from build123d import *

# Parameters (mm, degrees)
F0_R     = 1.1684
F1_DEPTH = 1.1811
F3_DEPTH = 4.7244
F5_DEPTH = 3.4798
F7_DEPTH = 4.4069


with BuildPart() as f1:
    # F0 (on Top) → F1 (new body, symmetric)
    with BuildSketch(Plane.XY):
        with BuildLine():
            Line((16.6497, 4.4577), (-16.6497, 4.4577))
            ThreePointArc((-16.6497, 4.4577), (-17.763252, 3.996452), (-18.2245, 2.8829))
            Line((-18.2245, 2.8829), (-18.2245, -2.8829))
            ThreePointArc((-18.2245, -2.8829), (-17.763252, -3.996452), (-16.6497, -4.4577))
            Line((-16.6497, -4.4577), (16.6497, -4.4577))
            ThreePointArc((16.6497, -4.4577), (17.763252, -3.996452), (18.2245, -2.8829))
            Line((18.2245, -2.8829), (18.2245, 2.8829))
            ThreePointArc((18.2245, 2.8829), (17.763252, 3.996452), (16.6497, 4.4577))
        make_face()
        with Locations((-15.4305, 0)):
            Circle(F0_R, mode=Mode.SUBTRACT)
        with Locations((15.4305, 0)):
            Circle(F0_R, mode=Mode.SUBTRACT)
    extrude(amount=F1_DEPTH, both=True)

    # F2 (on face) → F3 (join)
    with BuildSketch(Plane.XY.offset(1.1811)):
        with BuildLine():
            Line((-11.10602, -2.8956), (11.107478, -2.8956))
            ThreePointArc((11.107478, -2.8956), (12.464371, -2.120071), (12.484829, -0.557322))
            Line((12.484829, -0.557322), (11.020566, 2.084278))
            ThreePointArc((11.020566, 2.084278), (10.442486, 2.677694), (9.643215, 2.8956))
            Line((9.643215, 2.8956), (-9.641757, 2.8956))
            ThreePointArc((-9.641757, 2.8956), (-10.441029, 2.677694), (-11.019108, 2.084278))
            Line((-11.019108, 2.084278), (-12.483371, -0.557322))
            ThreePointArc((-12.483371, -0.557322), (-12.462914, -2.120071), (-11.10602, -2.8956))
        make_face()
    extrude(amount=F3_DEPTH)

    # F4 (on face) → F5 (join)
    with BuildSketch(Plane(origin=(0, 0, -1.1811), x_dir=(1, 0, 0), z_dir=(0, 0, -1))):
        with BuildLine():
            Line((12.7, 2.8956), (-12.7, 2.8956))
            ThreePointArc((-12.7, 2.8956), (-13.149013, 2.709613), (-13.335, 2.2606))
            Line((-13.335, 2.2606), (-13.335, -2.2606))
            ThreePointArc((-13.335, -2.2606), (-13.149013, -2.709613), (-12.7, -2.8956))
            Line((-12.7, -2.8956), (12.7, -2.8956))
            ThreePointArc((12.7, -2.8956), (13.149013, -2.709613), (13.335, -2.2606))
            Line((13.335, -2.2606), (13.335, 2.2606))
            ThreePointArc((13.335, 2.2606), (13.149013, 2.709613), (12.7, 2.8956))
        make_face()
    extrude(amount=F5_DEPTH)

    # F6 (on face) → F7 (join)
    with BuildSketch(Plane.XY.offset(5.9055)):
        with BuildLine():
            Line((9.456193, 2.5781), (-9.454736, 2.5781))
            ThreePointArc((-9.454736, 2.5781), (-10.254007, 2.360194), (-10.832087, 1.766778))
            Line((-10.832087, 1.766778), (-12.195227, -0.692392))
            ThreePointArc((-12.195227, -0.692392), (-12.178729, -1.952674), (-11.08446, -2.5781))
            Line((-11.08446, -2.5781), (11.085917, -2.5781))
            ThreePointArc((11.085917, -2.5781), (12.180186, -1.952674), (12.196684, -0.692392))
            Line((12.196684, -0.692392), (10.833544, 1.766778))
            ThreePointArc((10.833544, 1.766778), (10.255464, 2.360194), (9.456193, 2.5781))
        make_face()
    extrude(amount=F7_DEPTH)


solid = f1.part
Work out the finished part from the listing and answer in its coordinate system (mm). A direction names the side the tool comes from. Round coordinates to 2 decimals unless told otherwise and drop trailing zeros. Write each loop counter-clockwise with the first axis right and the second up, starting at its lowest first coordinate (ties: lowest second). Pieces come first, ordered by that corner, then holes. Notation, with made-up numbers: (0.25, -2.5) - (6.25, -2.5) arc R9 cw to (6.25, 2.5) - close; hole circle Ø9 at (15, 38.25). An arc over 180 degrees is marked (long way). Answer in a Markdown table with one row per item. Add a question column.
1. A cutting plane is placed at D-D, the plane x = 16. Determine the outline of the cut face in (y, z), and give its area (3 significant figures).
2. Find the intervals of material crossed by line 1 along Y through (x, z) = (-5.5, 6.75); line 2 along Z through (x, y) = (12, 2.25); line 3 along Z through (x, y) = (14.5, -2.75), in increasing order. Write a range as from..to.
3. A cutting plane is placed at C-C, the plane x = 6. Determine the outline of the cut face in (y, z).
4. A cutting plane is placed at A-A, the plane z = 8. Determine the outline of the cut face in (x, y), and give its area (3 significant figures).
5. A cutting plane is placed at B-B, the plane y = 0.75. Count the separate pieces of the cut face and the enclosed holes in it, and give its area (3 significant figures).
6. Given pin 1 (1 mm diameter, centred on y = -2, z = 7, fed in from +X); pin 2 (3 mm diameter, centred on y = 3, z = 8, fed in from -X); pin 3 (1.7 mm diameter, centred on y = 1, z = -2.5, fed in from +X) (3 decimals), each flat-ended and moving along its own axis, determine where each tip first touches the part or whether it passes through.
7. For faces 1 (the cylindrical face through (12.453, -2.14, 3.51)), 2 (the flat face through (11.525, 0.52, 8.078)), 3 (the flat face through (0, 2.578, 8)), 4 (the flat face through (-11.74, 0.78, 3.51)), determine the directions among +Z, -Z, +X, -X, +Y, -Y from which every point of the face is accessible in a straight line to the end or side of a thin tool.
8. The mould has two halves that part along Y. Classify faces 5 (the flat face through (0, -2.578, 8)), 6 (the cylindrical face through (14.503, -0.711, -0.017)), 7 (the flat face through (-11.504, 0.554, 8.078)): +Y half, -Y half, draft (parallel to the pull), parting line (faces both ways), or undercut.
Worked out:
| question | item | result |
|---|---|---|
| 1 | outline | (-4.46, -1.18) - (-1.02, -1.18) - (-1.02, 1.18) - (-4.46, 1.18) - close; (1.02, -1.18) - (4.46, -1.18) - (4.46, 1.18) - (1.02, 1.18) - close |
| 1 | area | 16.2 mm^2 |
| 2 | line 1 | -2.58..2.58 |
| 2 | line 2 | -4.66..1.18 |
| 2 | line 3 | -1.18..1.18 |
| 3 | outline | (-4.46, -1.18) - (-2.9, -1.18) - (-2.9, -4.66) - (2.9, -4.66) - (2.9, -1.18) - (4.46, -1.18) - (4.46, 1.18) - (2.9, 1.18) - (2.9, 5.91) - (2.58, 5.91) - (2.58, 10.31) - (-2.58, 10.31) - (-2.58, 5.91) - (-2.9, 5.91) - (-2.9, 1.18) - (-4.46, 1.18) - close |
| 4 | outline | (-12.2, -0.69) arc R1.27 ccw to (-11.08, -2.58) - (11.09, -2.58) arc R1.27 ccw to (12.2, -0.69) - (10.83, 1.77) arc R1.57 ccw to (9.46, 2.58) - (-9.45, 2.58) arc R1.57 ccw to (-10.83, 1.77) - close |
| 4 | area | 119 mm^2 |
| 5 | separate pieces | 3 |
| 5 | enclosed holes | 0 |
| 5 | area | 382 mm^2 |
| 6 | pin 1 | x = 12.34 |
| 6 | pin 2 | x = -10.98 |
| 6 | pin 3 | x = 13.335 |
| 7 | face 1 | +Z, +X |
| 7 | face 2 | +Z, +X, +Y |
| 7 | face 3 | +Z, +X, -X, +Y |
| 7 | face 4 | +Z, -X, +Y |
| 8 | face 5 | -Y half |
| 8 | face 6 | undercut |
| 8 | face 7 | +Y half |
